from build123d import *

# Parameters (mm, degrees)
CROQUIS1_R              = 12.7
SALIENTE_EXTRUIR1_DEPTH = 25.4
CROQUIS2_R              = 9.525
SALIENTE_EXTRUIR2_DEPTH = 50.8
REDONDEO1_R             = 1
REDONDEO2_R             = 1
CHAFL_N1_SIZE           = 1
CHAFL_N2_SIZE           = 1


with BuildPart() as part:
    # Croquis1 → Saliente-Extruir1 (new body, symmetric)
    with BuildSketch(Plane(origin=(0, 0, 0), x_dir=(0, 0, -1), z_dir=(1, 0, 0))):
        Circle(CROQUIS1_R)
    extrude(amount=SALIENTE_EXTRUIR1_DEPTH, both=True)

    # Croquis2 → Saliente-Extruir2 (add)
    with BuildSketch(Plane(origin=(25.4, 0, 0), x_dir=(0, 0, -1), z_dir=(1, 0, 0))):
        Circle(CROQUIS2_R)
    saliente_extruir2 = extrude(amount=SALIENTE_EXTRUIR2_DEPTH)

    # Redondeo1
    redondeo1_edges = [part.edges().sort_by_distance(p)[0] for p in [
        (25.4, 0, 9.525),
    ]]
    fillet(redondeo1_edges, radius=REDONDEO1_R)

    # Simetría3: Saliente-Extruir2 across plane
    add(saliente_extruir2.mirror(Plane(origin=(0, 0, 0), x_dir=(0, 0, 1), z_dir=(1, 0, 0))))

    # Redondeo2
    redondeo2_edges = [part.edges().sort_by_distance(p)[0] for p in [
        (-25.4, 0, 9.525),
    ]]
    fillet(redondeo2_edges, radius=REDONDEO2_R)

    # Chaflán1
    chafl_n1_edges = [part.edges().sort_by_distance(p)[0] for p in [
        (-76.2, 0, 9.525),
        (76.2, 0, 9.525),
    ]]
    chamfer(chafl_n1_edges, length=CHAFL_N1_SIZE)

    # Chaflán2
    chafl_n2_edges = [part.edges().sort_by_distance(p)[0] for p in [
        (-25.4, 0, 12.7),
        (25.4, 0, 12.7),
    ]]
    chamfer(chafl_n2_edges, length=CHAFL_N2_SIZE)


solid = part.part
Verification items for the finished model (mm, model axes). A direction names the side the tool comes from. Coordinates: 2 decimals unless noted, no trailing zeros. Write each loop counter-clockwise with the first axis right and the second up, starting at its lowest first coordinate (ties: lowest second). Pieces come first, ordered by that corner, then holes. Notation, with made-up numbers: M -11.5,-15 L 38.5,-15 A11 cw 38.5,-9 Z; hole C 50,67.25 d6. An arc over 180 degrees is marked long. Use a Markdown table: item, result.
Q1. Sectioned sample at A-A, the plane y = 0. Record the boundary of the cut face in (x, z) (3 decimals), plus the area to 3 significant figures.
Reply:
| item | result |
|---|---|
| outline | M -76.2,-8.525 L -75.2,-9.525 L -26.4,-9.525 A1 cw -25.4,-10.525 L -25.4,-11.7 L -24.4,-12.7 L 24.4,-12.7 L 25.4,-11.7 L 25.4,-10.525 A1 cw 26.4,-9.525 L 75.2,-9.525 L 76.2,-8.525 L 76.2,8.525 L 75.2,9.525 L 26.4,9.525 A1 cw 25.4,10.525 L 25.4,11.7 L 24.4,12.7 L -24.4,12.7 L -25.4,11.7 L -25.4,10.525 A1 cw -26.4,9.525 L -75.2,9.525 L -76.2,8.525 Z |
| area | 3,220 mm² |
Q2. Set-up check for faces 1 (the face through (-25.4, 4, 10)), 2 (the face through (25.4, 4, 10)), 3 (the face through (0.34, -12.4, 2.75)): record each of +Z, -Z, +X, -X, +Y, -Y from which the full face is reachable in a straight line by a thin tool's end or side.
Reply:
| item | result |
|---|---|
| face 1 | -X |
| face 2 | +X |
| face 3 | +X, -X |
Q3. Go/stop test with flat-tipped pins: P1, Ø10, axis at x = 44.5, z = 6, coming from the +Y side; P2, Ø5, axis at y = -1.5, z = 8.5, coming from the +X side; P3, Ø3, axis at x = 29, z = -1.5, coming from the -Y side (3 decimals); P4, Ø8, axis at x = 42, z = -7.5, coming from the +Y side. Record where each tip stops, or that it passes through.
Reply:
| item | result |
|---|---|
| P1 | stops at y = 9.47 |
| P2 | stops at x = 76.2 |
| P3 | stops at y = -9.525 |
| P4 | stops at y = 8.86 |
Q4. Thickness scan on line 1 (Y direction, x = 5.5, z = 0.75); line 2 (X direction, y = 4.5, z = -9.5); line 3 (Z direction, x = 64.5, y = -3). Record the ranges inside material, lowest first.
Reply:
| item | result |
|---|---|
| line 1 | y = -12.68 to 12.68 |
| line 2 | x = -25.4 to 25.4 |
| line 3 | z = -9.04 to 9.04 |
Q5. Sectioned sample at C-C, the plane x = 41.5. Record the boundary of the cut face in (y, z) (3 decimals), plus the area to 3 significant figures.
Reply:
| item | result |
|---|---|
| outline | C 0,0 d19.05 |
| area | 285 mm² |
